For this review, take the finished solid that the model builds, in its own axes (mm). A direction names the side the tool comes from. Coordinates: 2 decimals unless noted, no trailing zeros. Order: outer loops, then holes, each group sorted by start corner. A loop starts at its lowest first (then second) coordinate and runs counter-clockwise, first axis right, second up. Notation, with made-up numbers: (-8, -25.75) -> (7, -25.75) arc R24 cw to (7, -15.75) -> close; hole circle Ø7 at (65.5, 73). An arc over 180 degrees is marked (long way). Return JSON: item names as keys, results as strings. Group by question number.
Item 1: Insertion check: pin 1 (0.7 mm diameter, centred on x = 1, y = 12, fed in from +Z); pin 2 (0.7 mm diameter, centred on x = 1.5, y = 17.5, fed in from -Z); pin 3 (0.7 mm diameter, centred on y = 12.5, z = 1, fed in from +X). Each pin has a flat end and moves straight along its axis. Give the tip position at first contact, or say it passes through.
Item 2: Take a section at A-A (y = 13.5). Write out the cut boundary in (x, z).
Item 3: For line 1 along Z through (x, y) = (0.1, 11.5); line 2 along X through (y, z) = (5.5, 1.75), list the stretches that pass through material, from the lowest coordinate up.
Item 4: Machinability: for faces 1 (the cylindrical face through (-0.01, 11.5, 2.25)), 2 (the flat face through (-1, 11, -0.8)), 3 (the flat face through (0.8, 11, 1)), 4 (the flat face through (-1, 11, 0.8)), 5 (the flat face through (1, 11, -0.8)), which of the approach directions +Z, -Z, +X, -X, +Y, -Y give a long, thin tool a straight path to every point of the face, cutting with its end or side? Answer none if there is none.
```python
from build123d import *

# Parameters (mm, degrees)
BOSS_EXTRUDE1_DEPTH = 23.3
FILLET1_R           = 1
FILLET2_R           = 1
FILLET3_R           = 1
FILLET4_R           = 1
FILLET20_R          = 1
FILLET21_R          = 1
FILLET22_R          = 1
FILLET23_R          = 1


with BuildPart() as part:
    # Sketch1 → Boss-Extrude1 (new body)
    with BuildSketch(Plane(origin=(0, 0, 0), x_dir=(1, 0, 0), z_dir=(0, 1, 0))):
        with BuildLine():
            Line((-0.8, -0.8), (-0.8, -2.102974084))
            ThreePointArc((-0.8, -2.102974084), (0, -2.25), (0.8, -2.102974084))
            Line((0.8, -2.102974084), (0.8, -0.8))
            Line((0.8, -0.8), (2.102974084, -0.8))
            ThreePointArc((2.102974084, -0.8), (2.25, 0), (2.102974084, 0.8))
            Line((2.102974084, 0.8), (0.8, 0.8))
            Line((0.8, 0.8), (0.8, 2.102974084))
            ThreePointArc((0.8, 2.102974084), (0, 2.25), (-0.8, 2.102974084))
            Line((-0.8, 2.102974084), (-0.8, 0.8))
            Line((-0.8, 0.8), (-2.102974084, 0.8))
            ThreePointArc((-2.102974084, 0.8), (-2.25, 0), (-2.102974084, -0.8))
            Line((-2.102974084, -0.8), (-0.8, -0.8))
        make_face()
    extrude(amount=BOSS_EXTRUDE1_DEPTH)

    # Fillet1
    fillet1_edges = [part.edges().sort_by_distance(p)[0] for p in [
        (-2.25, 0, 0),
    ]]
    fillet(fillet1_edges, radius=FILLET1_R)

    # Fillet2
    fillet2_edges = [part.edges().sort_by_distance(p)[0] for p in [
        (0, 0, 2.25),
    ]]
    fillet(fillet2_edges, radius=FILLET2_R)

    # Fillet3
    fillet3_edges = [part.edges().sort_by_distance(p)[0] for p in [
        (2.25, 0, 0),
    ]]
    fillet(fillet3_edges, radius=FILLET3_R)

    # Fillet4
    fillet4_edges = [part.edges().sort_by_distance(p)[0] for p in [
        (0, 0, -2.25),
    ]]
    fillet(fillet4_edges, radius=FILLET4_R)

    # Fillet20
    fillet20_edges = [part.edges().sort_by_distance(p)[0] for p in [
        (2.25, 23.3, 0),
    ]]
    fillet(fillet20_edges, radius=FILLET20_R)

    # Fillet21
    fillet21_edges = [part.edges().sort_by_distance(p)[0] for p in [
        (0, 23.3, 2.25),
    ]]
    fillet(fillet21_edges, radius=FILLET21_R)

    # Fillet22
    fillet22_edges = [part.edges().sort_by_distance(p)[0] for p in [
        (-2.25, 23.3, 0),
    ]]
    fillet(fillet22_edges, radius=FILLET22_R)

    # Fillet23
    fillet23_edges = [part.edges().sort_by_distance(p)[0] for p in [
        (0, 23.3, -2.25),
    ]]
    fillet(fillet23_edges, radius=FILLET23_R)


solid = part.part
```
Findings below:
{
 "1": {"pin 1": "stops at z = 2.15", "pin 2": "stops at z = -0.8", "pin 3": "stops at x = 2.15"},
 "2": {"outline": "(-2.1, -0.8) -> (-0.8, -0.8) -> (-0.8, -2.1) arc R2.25 ccw to (0.8, -2.1) -> (0.8, -0.8) -> (2.1, -0.8) arc R2.25 ccw to (2.1, 0.8) -> (0.8, 0.8) -> (0.8, 2.1) arc R2.25 ccw to (-0.8, 2.1) -> (-0.8, 0.8) -> (-2.1, 0.8) arc R2.25 ccw to start"},
 "3": {"line 1": "z = -2.25 to 2.25", "line 2": "x = -0.8 to 0.8"},
 "4": {"face 1": "+Z, +Y, -Y", "face 2": "-Z, -X, +Y, -Y", "face 3": "+Z, +X, +Y, -Y", "face 4": "+Z, -X, +Y, -Y", "face 5": "-Z, +X, +Y, -Y"}
}
